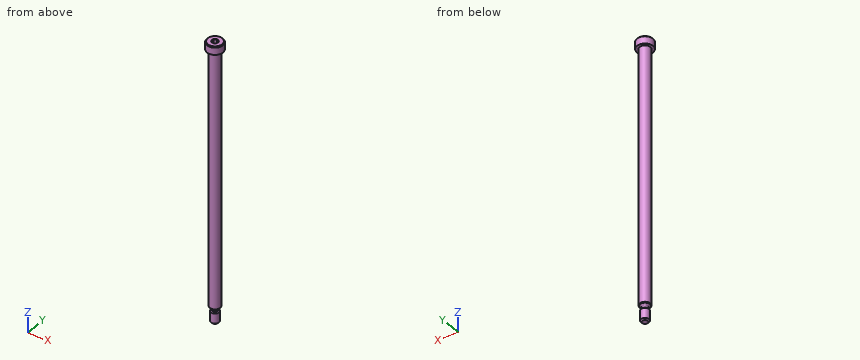
```python
from build123d import *

# Parameters (mm, degrees)
CUT_EXTRUDE1_DEPTH = 3.571875


with BuildPart() as part:
    # Sketch4 → Revolve1 (revolve)
    with BuildSketch(Plane(origin=(0, 0, 0), x_dir=(0, 0, -1), z_dir=(1, 0, 0)), mode=Mode.PRIVATE) as revolve1_sk:
        Polygon((-78.58125, 4.7625), (-82.8675, 4.7625), (-83.34375, 4.28625), (-83.34375, 0), (73.81875, 0), (73.81875, 2.921), (73.56475, 3.175), (-78.58125, 3.175), align=None)
    revolve(revolve1_sk.sketch.rotate(Axis((0, 0, 83.34375), (0, 0, -1)), 180), axis=Axis((0, 0, 83.34375), (0, 0, -1)))

    # Sketch5 → Cut-Extrude1 (cut)
    with BuildSketch(Plane.XY.offset(83.34375)):
        Polygon((1.5875, 0.916543552), (0, 1.833087105), (-1.5875, 0.916543552), (-1.5875, -0.916543552), (0, -1.833087105), (1.5875, -0.916543552), align=None)
    extrude(amount=-CUT_EXTRUDE1_DEPTH, mode=Mode.SUBTRACT)

    # Cut-Extrude4 cone 1 section (on through the dimple's axis) → Cut-Extrude4 (revolve, cut)
    with BuildSketch(Plane(origin=(0, 0, 83.34375), x_dir=(0, -1, 0), z_dir=(1, 0, 0))):
        Polygon((0, 0), (1.833087105, 0), (0, 1.833087105), align=None)
    revolve(axis=Axis((0, 0, 83.34375), (0, 0, -1)), mode=Mode.SUBTRACT)

    # Sketch7 → Revolve2 (revolve)
    with BuildSketch(Plane(origin=(0, 0, 0), x_dir=(0, 0, -1), z_dir=(1, 0, 0))):
        Polygon((73.81875, 2.413), (82.55, 2.413), (83.34375, 1.61925), (83.34375, 0), (73.81875, 0), align=None)
    revolve(axis=Axis((0, 0, -83.34375), (0, 0, 1)))

    # Sketch10 → Cut-Revolve1 (revolve, cut)
    with BuildSketch(Plane(origin=(0, 0, 0), x_dir=(0, 0, -1), z_dir=(1, 0, 0))):
        with BuildLine():
            Line((74.54265, 1.6891), (75.92695, 1.6891))
            Line((75.92695, 1.6891), (77.41285, 3.175))
            Line((77.41285, 3.175), (73.81875, 3.175))
            Line((73.81875, 3.175), (73.81875, 2.413))
            ThreePointArc((73.81875, 2.413), (74.030775401, 1.901125401), (74.54265, 1.6891))
        make_face()
    revolve(axis=Axis((0, 0, -83.34375), (0, 0, 1)), mode=Mode.SUBTRACT)


solid = part.part
```
Source: CAD feature listing. Evaluate the final solid. Frame: model axes, mm. Give positions to 0.01 mm unless a question says otherwise; leave off trailing zeros. Order: outer loops, then holes, each group sorted by start corner. A loop starts at its lowest first (then second) coordinate and runs counter-clockwise, first axis right, second up.
(1) Material intervals for line 1 along Z through (x, y) = (-4, -1.5); line 2 along Z through (x, y) = (-2, -0.25); line 3 along X through (y, z) = (0.25, 36.5), sorted ascending.
(2) Contact query for flat-ended pins moving along their axis: P1, Ø1.5, axis at y = -0.5, z = -22.5, coming from the -X side (3 decimals); P2, Ø2, axis at x = -3.5, z = -15.5, coming from the -Y side; P3, Ø4, axis at y = 3, z = -31.5, coming from the -X side. Output: stop coordinate, or through.
(3) Section query A-A (z = 37.5). Return the cut outline in (x, y) (3 decimals).
Outcome:
1. line 1: z = 78.58 to 83.34
1. line 2: z = -82.95 to -76.25, -73.94 to 83.34
1. line 3: x = -3.17 to 3.17
2. P1: stops at x = -3.175
2. P2: stops at y = -1.96
2. P3: stops at x = -3.01
3. outline: circle Ø6.35 at (0, 0)
